Autodesk Inventor part; units mm, degrees
ref_plane "YZ Plane" through (0, 0, 0) normal (1, 0, 0) x (0, 1, 0)
ref_plane "XZ Plane" through (0, 0, 0) normal (0, 1, 0) x (-1, 0, 0)
ref_plane "XY Plane" through (0, 0, 0) normal (0, 0, 1) x (1, 0, 0)
sketch "Sketch1" plane through (0, 0, 0) normal (0, 0, 1) x (1, 0, 0)
  line L0 (0, 0) -> (25.4, 0)
  line L1 (25.4, 0) -> (25.4, 25.4)
  line L2 (25.4, 25.4) -> (0, 25.4)
  line L3 (0, 25.4) -> (0, 0)
  line L4 (1.5875, 1.5875) -> (23.8125, 1.5875)
  line L5 (23.8125, 1.5875) -> (23.8125, 23.8125)
  line L6 (23.8125, 23.8125) -> (1.5875, 23.8125)
  line L7 (1.5875, 23.8125) -> (1.5875, 1.5875)
  dimension "d0" = 25.4
  dimension "d1" = 25.4
  dimension "d2" = 1.5875
extrude "Extrusion1" add sketch "Sketch1" along normal blind 558.8
sketch "Sketch3" plane through (0, 25.4, 0) normal (0, 1, 0) x (1, 0, 0)
  line L0 (25.4, 0) -> (0, 0)
  line L1 (0, 0) -> (0, -558.8)
  line L2 (25.4, -558.8) -> (0, -558.8)
  line L3 (25.4, 0) -> (25.4, -558.8)
  point P0 (0, 0)
  point P1 (12.7, -279.4)
  dimension "d15" = 279.4
  dimension "d16" = 558.8
  dimension "d17" = 12.7
hole "Hole2" at (12.7, 25.4, 279.4) direction (0, -1, 0) diameter 6.35 end through all
properties part number "ScissorLiftBarMiddle" material "Aluminum 6061"
Work out the finished part from the listing and answer in its coordinate system (mm). A direction names the side the tool comes from. Round coordinates to 2 decimals unless told otherwise and drop trailing zeros. Write each loop counter-clockwise with the first axis right and the second up, starting at its lowest first coordinate (ties: lowest second). Pieces come first, ordered by that corner, then holes. Notation, with made-up numbers: (80.25, 68.25) -> (84.25, 68.25) arc R24 ccw to (84.25, 81.25) -> close; hole circle Ø1 at (-22, 60). An arc over 180 degrees is marked (long way). Write each question's results on one line, items separated by ' | '.
Item 1: Which of the six approach directions +Z, -Z, +X, -X, +Y, -Y give full straight-line access (tool end or side, diameter ignored) to faces 4 (the face through (13, 1.588, 275)), 5 (the face through (0, 13, 275))?
Result set:
face 4: +Z, -Z | face 5: +Z, -Z, -X, +Y, -Y
Item 2: A cutting plane is placed at B-B, the plane z = 488.5. Determine the outline of the cut face in (x, y).
Result set:
outline: (0, 0) -> (25.4, 0) -> (25.4, 25.4) -> (0, 25.4) -> close; hole (1.59, 1.59) -> (23.81, 1.59) -> (23.81, 23.81) -> (1.59, 23.81) -> close
Item 3: A cutting plane is placed at A-A, the plane y = 16.5. Determine the outline of the cut face in (x, z).
Result set:
outline: (0, 0) -> (1.59, 0) -> (1.59, 558.8) -> (0, 558.8) -> close; (23.81, 0) -> (25.4, 0) -> (25.4, 558.8) -> (23.81, 558.8) -> close
Item 4: The mould has two halves that part along X. Classify faces 1 (the face through (25.4, 13, 275)), 2 (the face through (1, 13, 558.8)), 3 (the face through (13, 23.812, 275)): +X half, -X half, draft (parallel to the pull), parting line (faces both ways), or undercut.
Result set:
face 1: +X half | face 2: draft | face 3: undercut
Item 5: Find the intervals of material crossed by line 1 along Y through (x, z) = (11, 464); line 2 along Z through (x, y) = (12.7, 24.4) (3 decimals), in increasing order. Write a range as [from, to].
Result set:
line 1: [0, 1.59], [23.81, 25.4] | line 2: [0, 276.225], [282.575, 558.8]
